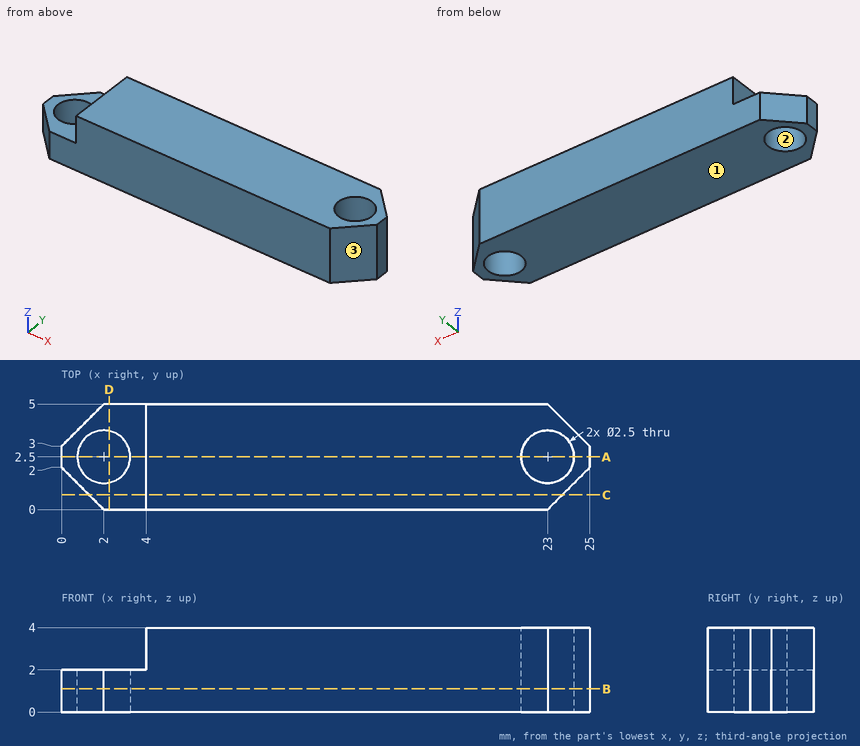
Geometry check sheet. Reference: drawing and pictorial views, mm from the part's lowest x, y, z. Round coordinates to 2 decimals unless told otherwise and drop trailing zeros. Write each loop counter-clockwise with the first axis right and the second up, starting at its lowest first coordinate (ties: lowest second). Pieces come first, ordered by that corner, then holes. Notation, with made-up numbers: (15, 81.5) -> (41, 81.5) arc R25 cw to (41, 113.5) -> close; hole circle Ø5 at (-2, 82). An arc over 180 degrees is marked (long way). Answer as CSV lines item,"result". Start each with the question number.
1) Go/stop test with flat-tipped pins: P1, Ø3, axis at x = 1, y = 3.5, coming from the +Z side; P2, Ø2, axis at x = 2, y = 2.5, coming from the +Z side; P3, Ø1, axis at y = 2.5, z = 3, coming from the -X side. Record where each tip stops, or that it passes through.
2) Section check C-C on y = 0.7. Enter the section's corners in (x, z), and give its area (3 significant figures).
3) Section check D-D on x = 2.25. Enter the section's corners in (y, z), and give its area (3 significant figures).
4) Section check A-A on y = 2.5. Enter the section's corners in (x, z), and give its area (3 significant figures).
5) Release check for a two-part mould opening along Y. For the marked faces 1, 2 and 3 record: pulls with the +Y half, pulls with the -Y half, needs draft (parallel to the pull), parting line crosses it, or undercut.
6) Material ranges on line 1 (Y direction, x = 22.25, z = 3.15); line 2 (Z direction, x = 3.25, y = 4.5); line 3 (X direction, y = 3.3, z = 3.5), recorded low to high. Write a range as from..to.
7) Section check B-B on z = 1.1. Enter the section's corners in (x, y).
Found:
1,P1,"stops at z = 2"
1,P2,"passes through"
1,P3,"stops at x = 4"
2,outline,"(1.3, 0) -> (23.7, 0) -> (23.7, 4) -> (4, 4) -> (4, 2) -> (1.3, 2) -> close"
2,area,"84.2 mm^2"
3,outline,"(0, 0) -> (1.28, 0) -> (1.28, 2) -> (0, 2) -> close; (3.72, 0) -> (5, 0) -> (5, 2) -> (3.72, 2) -> close"
3,area,"5.10 mm^2"
4,outline,"(0, 0) -> (0.75, 0) -> (0.75, 2) -> (0, 2) -> close; (3.25, 0) -> (21.75, 0) -> (21.75, 4) -> (4, 4) -> (4, 2) -> (3.25, 2) -> close; (24.25, 0) -> (25, 0) -> (25, 4) -> (24.25, 4) -> close"
4,area,"77.0 mm^2"
5,face 1,"needs draft"
5,face 2,"undercut"
5,face 3,"pulls with the -Y half"
6,line 1,"y = 0..1.5, 3.5..5"
6,line 2,"z = 0..2"
6,line 3,"x = 4..22.04, 23.96..24.7"
7,outline,"(0, 2) -> (2, 0) -> (23, 0) -> (25, 2) -> (25, 3) -> (23, 5) -> (2, 5) -> (0, 3) -> close; hole circle Ø2.5 at (2, 2.5); hole circle Ø2.5 at (23, 2.5)"
